```python
from build123d import *
from build123d import SkipClean  # not in build123d's __all__

# Parameters (mm, degrees)
F0_R     = 12.5
F1_DEPTH = 5
F2_DEPTH = 5.001
F3_DEPTH = 2.5


with BuildPart() as f1:
    # F0 (on Top) → F1 (new body, symmetric)
    with BuildSketch(Plane.XY):
        Circle(F0_R)
        with BuildLine():
            ThreePointArc((-2.8, -6.9577295147), (-4.1982139059, 6.2149014473), (7.5, 0))
            ThreePointArc((7.5, 0), (6.2149014473, -4.1982139059), (2.8, -6.9577295147))
            Line((2.8, -6.9577295147), (2.8, -10))
            Line((2.8, -10), (0, -10))
            Line((0, -10), (-2.8, -10))
            Line((-2.8, -10), (-2.8, -6.9577295147))
        make_face(mode=Mode.SUBTRACT)
        with BuildLine():
            ThreePointArc((2.8, -6.9577295147), (6.2149014473, -4.1982139059), (7.5, 0))
            ThreePointArc((7.5, 0), (-4.1982139059, 6.2149014473), (-2.8, -6.9577295147))
            ThreePointArc((-2.8, -6.9577295147), (0, -7.5), (2.8, -6.9577295147))
        make_face()
        with BuildLine():
            ThreePointArc((2.8, -6.9577295147), (0, -7.5), (-2.8, -6.9577295147))
            Line((-2.8, -6.9577295147), (-2.8, -10))
            Line((-2.8, -10), (0, -10))
            Line((0, -10), (2.8, -10))
            Line((2.8, -10), (2.8, -6.9577295147))
        make_face()
    extrude(amount=F1_DEPTH, both=True)

    # F0 (on Top) → F2 (cut, through all)
    with BuildSketch(Plane.XY):
        with BuildLine():
            ThreePointArc((2.8, -6.9577295147), (0, -7.5), (-2.8, -6.9577295147))
            Line((-2.8, -6.9577295147), (-2.8, -10))
            Line((-2.8, -10), (0, -10))
            Line((0, -10), (2.8, -10))
            Line((2.8, -10), (2.8, -6.9577295147))
        make_face()
        with BuildLine():
            ThreePointArc((2.8, -6.9577295147), (6.2149014473, -4.1982139059), (7.5, 0))
            ThreePointArc((7.5, 0), (-4.1982139059, 6.2149014473), (-2.8, -6.9577295147))
            ThreePointArc((-2.8, -6.9577295147), (0, -7.5), (2.8, -6.9577295147))
        make_face()
    extrude(amount=-F2_DEPTH, mode=Mode.SUBTRACT)

    # F0 (on Top) → F3 (join)
    with BuildSketch(Plane.XY):
        with BuildLine():
            ThreePointArc((2.8, -6.9577295147), (0, -7.5), (-2.8, -6.9577295147))
            Line((-2.8, -6.9577295147), (-2.8, -10))
            Line((-2.8, -10), (0, -10))
            Line((0, -10), (2.8, -10))
            Line((2.8, -10), (2.8, -6.9577295147))
        make_face()
    with SkipClean():  # cleaning this boolean's faces spoils the solid; the shape is the same uncleaned
        extrude(amount=-F3_DEPTH)


solid = f1.part
```
Input: part model. Units: mm. Frame: model coordinates. A direction names the side the tool comes from. Coordinates: 2 decimals unless noted, no trailing zeros. Order: outer loops, then holes, each group sorted by start corner. A loop starts at its lowest first (then second) coordinate and runs counter-clockwise, first axis right, second up. Notation, with made-up numbers: (48, 14.5) - (93, 14.5) arc R22 cw to (93, 30.5) - close; hole circle Ø2 at (0, -5.75). An arc over 180 degrees is marked (long way). Return JSON: item names as keys, results as strings.
Q1. Cut plane A-A (z = -4). Return loops of the section in (x, y), then the cut area to 3 significant figures.
The answers:
{"outline": "circle Ø25 at (0, 0); hole (-2.8, -10) - (2.8, -10) - (2.8, -6.96) arc R7.5 ccw (long way) to (-2.8, -6.96) - close", "area": "299 mm2"}
Q2. Access query for faces 1 (the flat face through (0, 0, 5)), 2 (the flat face through (-2.8, -8, -4)). Directions: +Z, -Z, +X, -X, +Y, -Y. A direction counts if a zero-diameter tool reaches every point of the face in a straight line with its end or side. Return the directions, or none.
The answers:
{"face 1": "+Z, +X, -X, +Y, -Y", "face 2": "-Z"}
Q3. Draft query along Y for faces 3 (the flat face through (0, -10, -4)), 4 (the flat face through (5, 6, -5)), 5 (the cylindrical face through (11.923, 3.755, 0.07)). Return one class per face: +Y half, -Y half, draft (parallel to the pull), parting line (faces both ways), or undercut.
The answers:
{"face 3": "undercut", "face 4": "draft", "face 5": "parting line"}
Q4. Cut plane C-C (x = 0). Return loops of the section in (y, z).
The answers:
{"outline": "(-12.5, -5) - (-10, -5) - (-10, -2.5) - (-7.5, -2.5) - (-7.5, 0) - (7.5, 0) - (7.5, -5) - (12.5, -5) - (12.5, 5) - (-12.5, 5) - close"}
Q5. Ray query, probe 1 along Y at (x, z) = (0, -1.1); probe 2 along Y at (x, z) = (0, -3.8); probe 3 along X at (y, z) = (0.25, 2.25). Return the intervals inside material, ascending.
The answers:
{"probe 1": "y = -12.5 to -7.5, 7.5 to 12.5", "probe 2": "y = -12.5 to -10, 7.5 to 12.5", "probe 3": "x = -12.5 to 12.5"}
Q6. First-contact query: pin 1 (4 mm diameter, centred on x = 9.5, z = -0.5, fed in from +Y); pin 2 (1.5 mm diameter, centred on x = -5, z = -0.5, fed in from -Y); pin 3 (2 mm diameter, centred on x = -9.5, z = -3, fed in from +Y). Flat tips, straight axial feed; report the tip coordinate or a pass-through.
The answers:
{"pin 1": "stops at y = 10", "pin 2": "stops at y = -11.76", "pin 3": "stops at y = 9.17"}
Q7. Cut plane D-D (z = 3.5). Return loops of the section in (x, y), then the cut area to 3 significant figures.
The answers:
{"outline": "circle Ø25 at (0, 0)", "area": "491 mm2"}
Q8. Cut plane B-B (y = -3.5). Return loops of the section in (x, z).
The answers:
{"outline": "(-12, -5) - (-6.63, -5) - (-6.63, 0) - (6.63, 0) - (6.63, -5) - (12, -5) - (12, 5) - (-12, 5) - close"}
